from build123d import *

# Parameters (mm, degrees)
F0_W     = 362
F0_H     = 10
F0_H_2   = 32.5
F1_DEPTH = 13
F2_DEPTH = 23
F3_DEPTH = 63
F4_D     = 9
F5_D     = 11
F6_D     = 10
F8_DEPTH = 349.501
F9_D     = 25
F10_R    = 2


with BuildPart() as f1:
    # F0 (on Top) → F1 (new body)
    with BuildSketch(Plane.XY):
        Polygon((0, 116), (0, 0), (0, -116), (50, -116), (50, -50), (40, -50), (40, 0), (40, 50), (50, 50), (50, 116), align=None)
        Polygon((0, 148.5), (0, 116), (50, 116), (362, 116), (362, 148.5), align=None)
        Polygon((50, -116), (0, -116), (0, -148.5), (362, -148.5), (362, -116), align=None)
        with Locations((181, 153.5)):
            Rectangle(F0_W, F0_H)
        with Locations((181, -153.5)):
            Rectangle(F0_W, F0_H)
        with Locations((181, 174.75)):
            Rectangle(F0_W, F0_H_2)
        Polygon((50, 0), (50, 50), (40, 50), (40, 0), (40, -50), (50, -50), align=None)
        with Locations((181, -174.75)):
            Rectangle(F0_W, F0_H_2)
    extrude(amount=-F1_DEPTH)

    # F0 (on Top) → F2 (join)
    with BuildSketch(Plane.XY):
        Polygon((50, 0), (50, 50), (40, 50), (40, 0), (40, -50), (50, -50), align=None)
    extrude(amount=-F2_DEPTH)

    # F0 (on Top) → F3 (join)
    with BuildSketch(Plane.XY):
        with Locations((181, 153.5)):
            Rectangle(F0_W, F0_H)
        with Locations((181, -153.5)):
            Rectangle(F0_W, F0_H)
    extrude(amount=F3_DEPTH)

    # F4 (through all)
    with Locations(Plane.XY):
        with Locations((236, 171.5), (306, 171.5), (346, 171.5), (236, 133.5), (306, 133.5), (346, 133.5), (236, -171.5), (306, -171.5), (346, -171.5), (236, -133.5), (306, -133.5), (346, -133.5)):
            Hole(F4_D / 2)

    # F5 (through all)
    with Locations(Plane.XY):
        with Locations((10, 130), (30, 75), (10, -130), (10, 0), (30, -75)):
            Hole(F5_D / 2)

    # F6 (through all)
    with Locations(Plane.XY):
        with Locations((27, 50), (27, -50)):
            Hole(F6_D / 2)

    # F7 (on face) → F8 (cut, through all)
    with BuildSketch(Plane.XZ.offset(158.5)):
        Polygon((50, 63), (0, 63), (0, 0), align=None)
        Polygon((312, 63), (362, 0), (362, 63), align=None)
    extrude(amount=-F8_DEPTH, mode=Mode.SUBTRACT)

    # F9 (through all)
    with Locations(Plane.XZ.offset(158.5)):
        with Locations((77, 25), (122, 25), (167, 25), (212, 25), (257, 25), (302, 25)):
            Hole(F9_D / 2)

    # F10
    f10_edges = [f1.edges().sort_by_distance(p)[0] for p in [
        (362, -191, -6.5),
        (362, 116, -6.5),
        (362, -116, -6.5),
        (362, 191, -6.5),
        (0, -191, -6.5),
        (0, 191, -6.5),
    ]]
    fillet(f10_edges, radius=F10_R)


solid = f1.part
Could you check a few things on this model? Use its own coordinates, in mm. A direction names the side the tool comes from. Coordinates: 2 decimals unless noted, no trailing zeros. Write each loop counter-clockwise with the first axis right and the second up, starting at its lowest first coordinate (ties: lowest second). Pieces come first, ordered by that corner, then holes. Notation, with made-up numbers: (48, 71) - (99, 71) arc R25 cw to (99, 95) - close; hole circle Ø4 at (82.5, 24.5). An arc over 180 degrees is marked (long way). Write item = value, one per line.
1) For faces 4 (the flat face through (45, 50, -18)), 5 (the flat face through (178.5, -158.5, 31.1)), 6 (the flat face through (40, 1, -18)), 7 (the flat face through (178, 175, 0)), which set-ups out of +Z, -Z, +X, -X, +Y, -Y let a thin tool reach every point of the face, with its end or its side?
Result set:
face_4 = -Z, +X, -X, +Y
face_5 = +Z, +X, -X, -Y
face_6 = -Z, -X, +Y, -Y
face_7 = +Z, +X, -X, +Y
2) Suppose I cut it at A-A on x = 346. State how many separate pieces and enclosed holes the cut face has, plus the area to 3 significant figures.
Result set:
separate_pieces = 6
enclosed_holes = 0
area = 1,890 mm2
3) Suppose I cut it at B-B on y = 75. Please give me the cut outline in (x, z).
Result set:
outline = (0, -13) - (24.5, -13) - (24.5, 0) - (0, 0) - close; (35.5, -13) - (50, -13) - (50, 0) - (35.5, 0) - close
4) We'd pull the mould along Y, two halves only. Please class faces 1 (the cylindrical face through (79.71, 153.57, 12.797)), 2 (the flat face through (45, -50, -18)), 3 (the flat face through (207, -116, -6)): +Y half, -Y half, draft (parallel to the pull), parting line (faces both ways), or undercut.
Result set:
face_1 = draft
face_2 = -Y half
face_3 = undercut
5) Suppose I cut it at D-D on z = 48.5. Please give me the cut outline in (x, y).
Result set:
outline = (38.49, -158.5) - (323.51, -158.5) - (323.51, -148.5) - (38.49, -148.5) - close; (38.49, 148.5) - (323.51, 148.5) - (323.51, 158.5) - (38.49, 158.5) - close
6) Will these pins go through, and if not, where does the flat tip stop? pin 1 Ø6 at (x, z) = (231.5, 8) entering from -Y; pin 2 Ø8 at (x, z) = (121, 46.5) entering from +Y; pin 3 Ø14.5 at (x, y) = (236, -171.5) entering from -Z.
Result set:
pin_1 = -158.5
pin_2 = 158.5
pin_3 = -13
7) Please list where these lines run through material, in increasing order: line 1 (Z direction, x = 77, y = -155.5); line 2 (X direction, y = -171, z = -8); line 3 (Y direction, x = 36, z = 30). Write a range as [from, to].
Result set:
line_1 = [-13, 12.5], [37.5, 63]
line_2 = [0, 231.53], [240.47, 301.53], [310.47, 341.53], [350.47, 362]
line_3 = [-158.5, -148.5], [148.5, 158.5]
8) Suppose I cut it at C-C on x = 187.5. Please give me the cut outline in (y, z).
Result set:
outline = (-191, -13) - (-116, -13) - (-116, 0) - (-148.5, 0) - (-148.5, 63) - (-158.5, 63) - (-158.5, 0) - (-191, 0) - close; (116, -13) - (191, -13) - (191, 0) - (158.5, 0) - (158.5, 63) - (148.5, 63) - (148.5, 0) - (116, 0) - close
